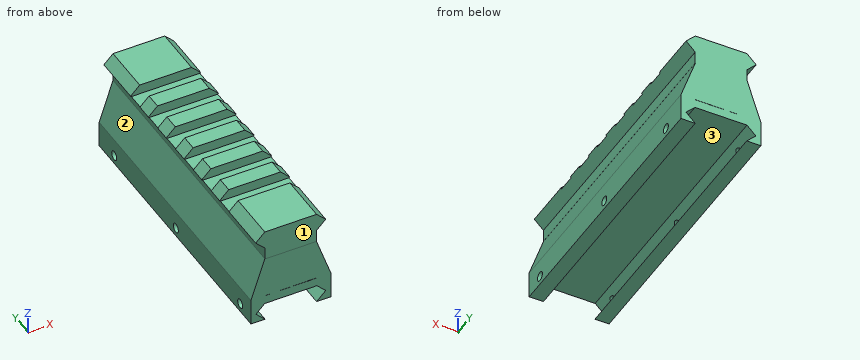
from build123d import *

# Parameters (mm, degrees)
F1_DEPTH       = 85.25
F2_W           = 55.8218845766
F2_H           = 5.25
F3_DEPTH       = 3
F5_DEPTH       = 85.2424
F8_D           = 2.794
F8_DEPTH       = 12.7
F8_TIP         = 0.8394022848
F8_ON_F7_D     = 2.794
F8_ON_F7_DEPTH = 12.7
F8_ON_F7_TIP   = 0.8394022848


with BuildPart() as f1:
    # F0 (on Front) → F1 (new body)
    with BuildSketch(Plane.XZ):
        Polygon((0, 3.79), (0, 0), (15.67, 0), (15.67, 3.79), (18.435, 6.555), (15.67, 9.32), (0, 9.32), (-2.765, 6.555), align=None)
    extrude(amount=F1_DEPTH)

    # F2 (on face) → F3 (cut)
    with BuildSketch(Plane.XY.offset(9.32)):
        with Locations((8.2114636898, -17.625)):
            Rectangle(F2_W, F2_H)
        with Locations((8.2114636898, -27.625)):
            Rectangle(F2_W, F2_H)
        with Locations((8.2114636898, -37.625)):
            Rectangle(F2_W, F2_H)
        with Locations((8.2114636898, -47.625)):
            Rectangle(F2_W, F2_H)
        with Locations((8.2114636898, -57.625)):
            Rectangle(F2_W, F2_H)
        with Locations((8.2114636898, -67.625)):
            Rectangle(F2_W, F2_H)
    extrude(amount=-F3_DEPTH, mode=Mode.SUBTRACT)

    # F4 (on Front) → F5 (join)
    with BuildSketch(Plane.XZ):
        Polygon((0.0019754424, -12.6376101786), (15.6015763059, -12.5601905993), (15.6015763059, 0), (15.6015763059, 0.1199992985), (0.0019754424, 0.1199992985), (0.0019754424, -2.5521272328), align=None)
        Polygon((18.4492052038, -17.9727599025), (15.6827729632, -20.7406985573), (19.9911782954, -20.7406985573), (19.9911782954, -12.5384053536), (15.6015763059, -12.5601905993), (15.6015763059, -12.6442629844), (0.0019754424, -12.6442629844), (0.0019754424, -12.6376101786), (-4.1879916127, -12.658404652), (-4.1879916127, -20.7361024804), (0.0811966573, -20.7361024804), (-2.6852355834, -17.9681638256), (0, -15.2933802456), (15.7593555839, -15.2933802456), align=None)
        Polygon((15.6015763059, -12.5601905993), (19.9911782954, -12.5384053536), (15.6015763059, 0.1199992985), (15.6015763059, 0), align=None)
        Polygon((-4.1879916127, -12.658404652), (0.0019754424, -12.6376101786), (0.0019754424, -2.5521272328), (0.0019754424, 0.1199992985), align=None)
    extrude(amount=F5_DEPTH)

    # F8 (one way)
    with BuildSketch(Plane.YZ):
        with Locations((-79.1830047965, -18.0843956769), (-43.074503541, -18.0843956769), (-8.4564629942, -18.0843956769)):
            Circle(F8_D / 2)
    extrude(amount=-F8_DEPTH, mode=Mode.SUBTRACT)
    with Locations(Plane.YZ):
        with Locations((-79.1830047965, -18.0843956769), (-43.074503541, -18.0843956769), (-8.4564629942, -18.0843956769)):
            with Locations((0, 0, -(F8_DEPTH + F8_TIP / 2))):  # 118° drill point
                Cone(0, F8_D / 2, F8_TIP, mode=Mode.SUBTRACT)

    # F8 on F7
    with Locations(Plane.YZ.offset(19.9911782954)):
        with Locations((-79.1751816869, -18.0775541812), (-43.0787950754, -18.0775541812), (-8.4547195584, -18.0775541812)):
            Hole(F8_ON_F7_D / 2, depth=F8_ON_F7_DEPTH)
            with Locations((0, 0, -(F8_ON_F7_DEPTH + F8_ON_F7_TIP / 2))):  # 118° drill point
                Cone(0, F8_ON_F7_D / 2, F8_ON_F7_TIP, mode=Mode.SUBTRACT)


solid = f1.part
Geometry check sheet. Reference: the model listing, model coordinates, mm. Face numbers are marked on the shaded views. Round coordinates to 2 decimals unless told otherwise and drop trailing zeros. Order: outer loops, then holes, each group sorted by start corner. A loop starts at its lowest first (then second) coordinate and runs counter-clockwise, first axis right, second up. Notation, with made-up numbers: (36.5, 73.25) - (77.5, 73.25) arc R22 cw to (77.5, 99.25) - close; hole circle Ø10 at (38.25, 34.5). An arc over 180 degrees is marked (long way). One line per question, with ' | ' between items. Start each with the question number.
(1) Depth check by flat-ended pin: pin 1 Ø4 at (y, z) = (-69.5, -7) entering from +X; pin 2 Ø6.5 at (x, z) = (4.5, -9) entering from -Y; pin 3 Ø1.5 at (x, y) = (0.5, -26.5) entering from -Z; pin 4 Ø2.5 at (y, z) = (-79.18, -18.08) entering from -X. Enter the tip coordinate at first touch or a pass-through.
(2) Sectioned sample at A-A on z = 7.5. Record the cut outline in (x, y).
(3) Thickness scan on L1, parallel to Y at x = 10.5, z = -3.5; L2, parallel to X at y = -47.5, z = -6.5; L3, parallel to X at y = -61.5, z = -19. Record the ranges inside material, lowest first. Write a range as [from, to].
(4) Sectioned sample at D-D on y = -75.5. Record the cut outline in (x, z) (3 decimals), and give its area (3 significant figures).
(5) Release check for a two-part mould opening along X. For the marked faces 1, 2 and 3 record: released by +X, released by -X, zero draft, split by the parting line, or undercut.
Conclusion:
1) pin 1: stops at x = 18.76 | pin 2: stops at y = -85.24 | pin 3: stops at z = -20.74 | pin 4: passes through
2) outline: (-1.82, -85.25) - (17.49, -85.25) - (17.49, -70.25) - (-1.82, -70.25) - close; (-1.82, -65) - (17.49, -65) - (17.49, -60.25) - (-1.82, -60.25) - close; (-1.82, -55) - (17.49, -55) - (17.49, -50.25) - (-1.82, -50.25) - close; (-1.82, -45) - (17.49, -45) - (17.49, -40.25) - (-1.82, -40.25) - close; (-1.82, -35) - (17.49, -35) - (17.49, -30.25) - (-1.82, -30.25) - close; (-1.82, -25) - (17.49, -25) - (17.49, -20.25) - (-1.82, -20.25) - close; (-1.82, -15) - (17.49, -15) - (17.49, 0) - (-1.82, 0) - close
3) L1: y = [-85.24, 0] | L2: x = [-2.17, 17.9] | L3: x = [-4.19, -1.65], [17.42, 19.99]
4) outline: (-4.188, -20.736) - (0.081, -20.736) - (-2.685, -17.968) - (0, -15.293) - (15.759, -15.293) - (18.449, -17.973) - (15.683, -20.741) - (19.991, -20.741) - (19.991, -12.538) - (15.643, 0) - (15.67, 0) - (15.67, 3.79) - (18.435, 6.555) - (15.67, 9.32) - (0, 9.32) - (-2.765, 6.555) - (0, 3.79) - (0, 0.114) - (-4.188, -12.658) - close; hole (0.002, -12.644) - (15.602, -12.644) - (15.602, -12.56) - (0.002, -12.638) - close | area: 508 mm2
5) face 1: zero draft | face 2: released by -X | face 3: undercut
